Work out the finished part from the listing and answer in its coordinate system (mm). Coordinates: 2 decimals unless noted, no trailing zeros. Write each loop counter-clockwise with the first axis right and the second up, starting at its lowest first coordinate (ties: lowest second). Pieces come first, ordered by that corner, then holes. Notation, with made-up numbers: M 67.5,33 L 96.5,33 A29 ccw 96.5,57 Z; hole C 16.5,39 d9. An arc over 180 degrees is marked long. Answer as CSV lines item,"result". Start each with the question number.
(1) Flat-ended cylindrical pins translate along their axes: P1, Ø0.6, axis at x = 104, y = 30.5, coming from the -Z side; P2, Ø9, axis at x = 81.46, y = 30, coming from the -Z side; P3, Ø3, axis at x = 81.46, y = 45, coming from the -Z side. Find the tip coordinate at first contact, or state that the pin passes through.
(2) A cutting plane is placed at B-B on y = 45. Give the vertices of the cut face in (x, z).
(3) A cutting plane is placed at C-C on x = 73.5. Give the vertices of the cut face in (y, z).
(4) A cutting plane is placed at A-A on y = 22. Give the vertices of the cut face in (x, z), then the cut area to 3 significant figures.
(5) Find the intervals of material crossed by L1, parallel to Y at x = 82, z = 1.75; L2, parallel to Y at x = 80, z = 2.2; L3, parallel to X at y = 21, z = 1.55, in increasing order. Write a range as [from, to].
(6) A cutting plane is placed at D-D on y = 60. Give the vertices of the cut face in (x, z), then the cut area to 3 significant figures.
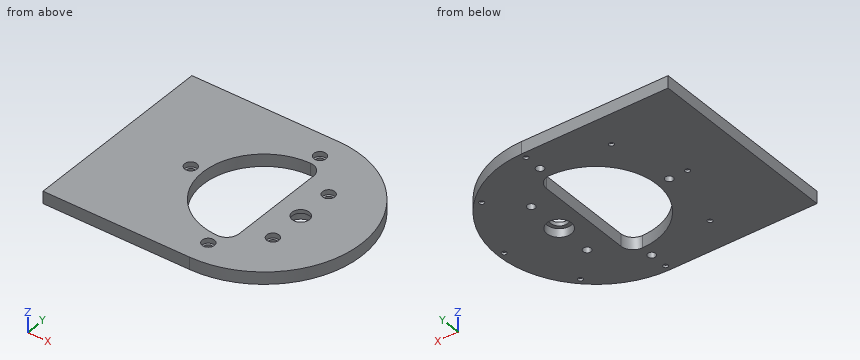
from build123d import *

# Parameters (mm, degrees)
EXTRUDE_1_DEPTH      = 5
CUT_EXTRUDE_2_DEPTH  = 10
SKETCH_4_R           = 5
CUT_EXTRUDE_3_DEPTH  = 3.5
SKETCH_8_R           = 1
CUT_EXTRUDE_7_DEPTH  = 1
SKETCH_10_R          = 2.5
CUT_EXTRUDE_8_DEPTH  = 2
SKETCH_9_R           = 1.6
CUT_EXTRUDE_9_DEPTH  = 3
SKETCH_11_R          = 3.5
CUT_EXTRUDE_10_DEPTH = 10


with BuildPart() as part:
    # 草图1 → 凸台-拉伸1 (new body)
    with BuildSketch(Plane.XY):
        with BuildLine():
            Line((66.457513111, 70), (6.457513111, 70))
            Line((6.457513111, 70), (6.457513111, -10))
            Line((6.457513111, -10), (66.457513111, -10))
            ThreePointArc((66.457513111, -10), (106.457513111, 30), (66.457513111, 70))
        make_face()
    extrude(amount=EXTRUDE_1_DEPTH)

    # 草图3 → 切除-拉伸2 (cut)
    with BuildSketch(Plane.XY):
        with BuildLine():
            Line((71.457513111, 35), (71.457513111, 50))
            ThreePointArc((71.457513111, 50), (69.993047017, 53.535533906), (66.457513111, 55))
            ThreePointArc((66.457513111, 55), (41.457513111, 30), (66.457513111, 5))
            ThreePointArc((66.457513111, 5), (69.993047017, 6.464466094), (71.457513111, 10))
            Line((71.457513111, 10), (71.457513111, 35))
        make_face()
    extrude(amount=CUT_EXTRUDE_2_DEPTH, mode=Mode.SUBTRACT)

    # 草图4 → 切除-拉伸3 (cut)
    with BuildSketch(Plane.XY):
        with Locations((81.457513111, 30)):
            Circle(SKETCH_4_R)
    extrude(amount=CUT_EXTRUDE_3_DEPTH, mode=Mode.SUBTRACT)

    # 草图8 → 切除-拉伸7 (cut)
    with BuildSketch(Plane.XY):
        with Locations((66.457513111, 67.5)):
            Circle(SKETCH_8_R)
        with Locations((92.974017405, 56.516504294)):
            Circle(SKETCH_8_R)
        with Locations((103.957513111, 30)):
            Circle(SKETCH_8_R)
        with Locations((92.974017405, 3.483495706)):
            Circle(SKETCH_8_R)
        with Locations((66.457513111, -7.5)):
            Circle(SKETCH_8_R)
        with Locations((39.941008816, 3.483495706)):
            Circle(SKETCH_8_R)
        with Locations((28.957513111, 30)):
            Circle(SKETCH_8_R)
        with Locations((39.941008816, 56.516504294)):
            Circle(SKETCH_8_R)
    extrude(amount=CUT_EXTRUDE_7_DEPTH, mode=Mode.SUBTRACT)

    # 草图10 → 切除-拉伸8 (cut)
    with BuildSketch(Plane.XY.offset(5)):
        with Locations((66.457513111, 60)):
            Circle(SKETCH_10_R)
        with Locations((81.457513111, 45)):
            Circle(SKETCH_10_R)
        with Locations((66.457513111, 0)):
            Circle(SKETCH_10_R)
        with Locations((36.457513111, 30)):
            Circle(SKETCH_10_R)
        with Locations((81.457513111, 15)):
            Circle(SKETCH_10_R)
    extrude(amount=-CUT_EXTRUDE_8_DEPTH, mode=Mode.SUBTRACT)

    # 草图9 → 切除-拉伸9 (cut)
    with BuildSketch(Plane.XY):
        with Locations((81.457513111, 45)):
            Circle(SKETCH_9_R)
        with Locations((66.457513111, 60)):
            Circle(SKETCH_9_R)
        with Locations((81.457513111, 15)):
            Circle(SKETCH_9_R)
        with Locations((66.457513111, 0)):
            Circle(SKETCH_9_R)
        with Locations((36.457513111, 30)):
            Circle(SKETCH_9_R)
    extrude(amount=CUT_EXTRUDE_9_DEPTH, mode=Mode.SUBTRACT)

    # 草图11 → 切除-拉伸10 (cut)
    with BuildSketch(Plane.XY.offset(5)):
        with Locations((81.457513111, 30)):
            Circle(SKETCH_11_R)
    extrude(amount=-CUT_EXTRUDE_10_DEPTH, mode=Mode.SUBTRACT)


solid = part.part
Here are the results:
1,P1,"stops at z = 1"
1,P2,"stops at z = 3.5"
1,P3,"passes through"
2,outline,"M 6.46,0 L 46.46,0 L 46.46,5 L 6.46,5 Z; M 71.46,0 L 79.86,0 L 79.86,3 L 78.96,3 L 78.96,5 L 71.46,5 Z; M 83.06,0 L 103.54,0 L 103.54,5 L 83.96,5 L 83.96,3 L 83.06,3 Z"
3,outline,"M -9.38,0 L 69.38,0 L 69.38,5 L -9.38,5 Z"
4,outline,"M 6.46,0 L 42.77,0 L 42.77,5 L 6.46,5 Z; M 71.46,0 L 105.65,0 L 105.65,5 L 71.46,5 Z"
4,area,"353 mm^2"
5,L1,"y = [-6.86, 13.49], [16.51, 25.03], [34.97, 43.49], [46.51, 66.86]"
5,L2,"y = [-7.64, 14.34], [15.66, 25.22], [34.78, 44.34], [45.66, 67.64]"
5,L3,"x = [6.46, 43.13], [71.46, 105.43]"
6,outline,"M 6.46,0 L 64.86,0 L 64.86,3 L 63.96,3 L 63.96,5 L 6.46,5 Z; M 68.06,0 L 92.92,0 L 92.92,5 L 68.96,5 L 68.96,3 L 68.06,3 Z"
6,area,"413 mm^2"
